The model under review builds one solid part; all positions refer to its coordinate system, in mm. A direction names the side the tool comes from. Coordinates: 2 decimals unless noted, no trailing zeros. Write each loop counter-clockwise with the first axis right and the second up, starting at its lowest first coordinate (ties: lowest second). Pieces come first, ordered by that corner, then holes. Notation, with made-up numbers: (55.5, 67.25) - (90.5, 67.25) arc R22 cw to (90.5, 76.25) - close; hole circle Ø4 at (67, 7). An arc over 180 degrees is marked (long way). Put each result on its own line as item: value. Start each with the question number.
Item 1: Consider section A-A on z = -11. Give the boundary of the cut face in (x, y).
Item 2: To check wall thickness, follow L1, parallel to Z at x = 5, y = 7.5; L2, parallel to X at y = 19.5, z = 8; L3, parallel to Z at x = 0, y = 5. State the ranges of each line that lie inside material, in increasing order. Write a range as [from, to].
Item 3: Consider section B-B on x = 17.5. Give the boundary of the cut face in (y, z), then the cut area to 3 significant figures.
Item 4: Consider section C-C on x = 0. Give the boundary of the cut face in (y, z), then the cut area to 3 significant figures.
Item 5: Mouldability with a two-part tool opening along Z and no side actions: class faces 1 (the face through (-2.32, 10.35, -13.61)), 2 (the face through (0, 21, -5)) as pulls with the +Z half, pulls with the -Z half, needs draft (parallel to the pull), parting line crosses it, or undercut.
Item 6: For pin 1 (1.5 mm diameter, centred on y = 7, z = 6, fed in from +X); pin 2 (3 mm diameter, centred on x = -15, y = 8, fed in from -Z); pin 3 (8 mm diameter, centred on x = -14.5, y = 14, fed in from +Z), all flat-tipped, find the tip position at first contact; note any pin that passes through.
Item 7: Consider section D-D on y = 9.75. State how many separate pieces and enclosed holes the cut face has, then the cut area to 3 significant figures.
Item 8: Machinability: for faces 3 (the face through (0, 0, -5)), 4 (the face through (-6.08, 10.35, -4.39)), which of the approach directions +Z, -Z, +X, -X, +Y, -Y give a long, thin tool a straight path to every point of the face, cutting with its end or side? Answer none if there is none.
Autodesk Inventor part; units mm, degrees
ref_plane "YZ Plane" through (0, 0, 0) normal (1, 0, 0) x (0, 1, 0)
ref_plane "XZ Plane" through (0, 0, 0) normal (0, 1, 0) x (-1, 0, 0)
ref_plane "XY Plane" through (0, 0, 0) normal (0, 0, 1) x (1, 0, 0)
sketch "Sketch1" plane through (0, 0, 0) normal (0, 1, 0) x (-1, 0, 0)
  circle A0 centre (0, 0) radius 4.5
  circle A1 centre (0, 0) radius 25
  circle A2 centre (0, 0) radius 7.5
  circle A3 centre (0, 0) radius 21
  line L0 (0, 0) -> (25, 0)
  line L1 (22.5, 2) -> (22.5, -2)
  line L2 (22.5, -2) -> (2.5, -2)
  line L3 (2.5, -2) -> (2.5, 2)
  line L4 (2.5, 2) -> (22.5, 2)
  line L5 (22.5, 2) -> (2.5, -2) construction
  line L6 (22.5, -2) -> (2.5, 2) construction
  line L7 (5.0508, 22.0168) -> (8.855, 20.7807)
  line L8 (-1.1296, 2.9957) -> (5.0508, 22.0168)
  line L9 (8.855, 20.7807) -> (2.6747, 1.7596)
  line L10 (2.6747, 1.7596) -> (-1.1296, 2.9957)
  line L11 (-19.3785, 11.6071) -> (-17.0273, 14.8432)
  line L12 (-3.1981, -0.1486) -> (-19.3785, 11.6071)
  line L13 (-17.0273, 14.8432) -> (-0.847, 3.0875)
  line L14 (-0.847, 3.0875) -> (-3.1981, -0.1486)
  line L15 (-17.0273, -14.8432) -> (-19.3785, -11.6071)
  line L16 (-0.847, -3.0875) -> (-17.0273, -14.8432)
  line L17 (-19.3785, -11.6071) -> (-3.1981, 0.1486)
  line L18 (-3.1981, 0.1486) -> (-0.847, -3.0875)
  line L19 (8.855, -20.7807) -> (5.0508, -22.0168)
  line L20 (2.6747, -1.7596) -> (8.855, -20.7807)
  line L21 (5.0508, -22.0168) -> (-1.1296, -2.9957)
  line L22 (-1.1296, -2.9957) -> (2.6747, -1.7596)
  point P0 (12.5, 0)
  point P1 (7.2284, -2)
  point P2 (20.9045, -2)
  point P3 (8.362, -19.2634)
  point P4 (4.1358, -6.2566)
  point P5 (7.2284, 2)
  point P6 (4.1358, 6.2566)
  point P7 (8.362, 19.2634)
  point P8 (20.9045, 2)
  point P9 (0.3316, 7.4927)
  point P10 (-4.6723, 5.8668)
  point P11 (-15.7366, 13.9054)
  point P12 (4.5577, 20.4994)
  point P13 (-4.6723, -5.8668)
  point P14 (0.3316, -7.4927)
  point P15 (4.5577, -20.4994)
  point P16 (-15.7366, -13.9054)
  point P17 (-7.0235, 2.6307)
  point P18 (-7.0235, -2.6307)
  point P19 (-18.0877, -10.6693)
  point P20 (-18.0877, 10.6693)
  dimension "d1" = 50
  dimension "d0" = 9
  dimension "d2" = 3
  dimension "d3" = 4
  dimension "d4" = 4
  dimension "d5" = 20
  dimension "d8" = 360
extrude "Extrusion1" add sketch "Sketch1" along normal blind 21 contours L0 A2 L2 A0 | A0 L4 A2 L0 | A0 L9 A2 L4 | L2 A2 L20 A0 | L0 A3 L2 A2 | A2 L4 A3 L0 | A0 L8 A2 L9 | L20 A2 L21 A0 | L0 L1 L2 A3 | A3 L4 L1 L0 | A0 L13 A2 L8 | A2 L8 A3 L9 | A1 | L21 A2 L16 A0 | L20 A3 L21 A2 | A0 L12 A2 L13 | A3 L8 L7 L9 | L16 A2 L17 A0 | L20 L19 L21 A3 | A0 L17 A2 L12 | A2 L12 A3 L13 | L16 A3 L17 A2 | A3 L12 L11 L13 | L16 L15 L17 A3
fillet "Fillet1" radius 2 4 edges at (-8.362, 10.5, 19.2634) (-20.9045, 10.5, 2) (-7.2284, 10.5, 2) (-4.1358, 10.5, 6.2566)
pattern_circular "Circular Pattern1" count 5 over 360 about axis through (0, 0, 0) along (0, 1, 0) of "Fillet1"
properties part number "8_21mm"
Report:
1. outline: (-22.45, 0) - (-17.89, 0) - (-17.89, 21) - (-22.45, 21) - close; (-5.68, 0) - (-1.47, 0) - (-1.47, 21) - (-5.68, 21) - close; (11.74, 0) - (22.45, 0) - (22.45, 21) - (11.74, 21) - close
2. L1: [-24.49, -20.4], [-6.34, 6.34], [20.4, 24.49]
2. L2: [-23.69, -19.42], [-4.7, -0.26], [7.61, 14.41], [19.42, 23.69]
2. L3: [-25, -21], [-7.79, -4.5], [4.5, 7.79], [21, 25]
3. outline: (0, -17.85) - (21, -17.85) - (21, -9.68) - (0, -9.68) - close; (0, 9.68) - (21, 9.68) - (21, 17.85) - (0, 17.85) - close
3. area: 343 mm²
4. outline: (0, -25) - (21, -25) - (21, -21) - (0, -21) - close; (0, -7.79) - (21, -7.79) - (21, -4.5) - (0, -4.5) - close; (0, 4.5) - (21, 4.5) - (21, 7.79) - (0, 7.79) - close; (0, 21) - (21, 21) - (21, 25) - (0, 25) - close
4. area: 306 mm²
5. face 1: undercut
5. face 2: needs draft
6. pin 1: x = 24.44
6. pin 2: z = -21.04
6. pin 3: z = 22.69
7. separate pieces: 1
7. enclosed holes: 6
7. area: 978 mm²
8. face 3: +Z, -Z, +X, -X, -Y
8. face 4: +Y, -Y
